Study the drawing (mm; zero at the part's minimum x, y, z) and answer. Round coordinates to 2 decimals unless told otherwise and drop trailing zeros. Write each loop counter-clockwise with the first axis right and the second up, starting at its lowest first coordinate (ties: lowest second). Pieces come first, ordered by that corner, then holes. Notation, with made-up numbers: (58.25, 75) -> (73.25, 75) arc R5 ccw to (73.25, 79) -> close; hole circle Ø4 at (63, 84.25). An arc over 180 degrees is marked (long way). Return JSON: item names as keys, results as strings.
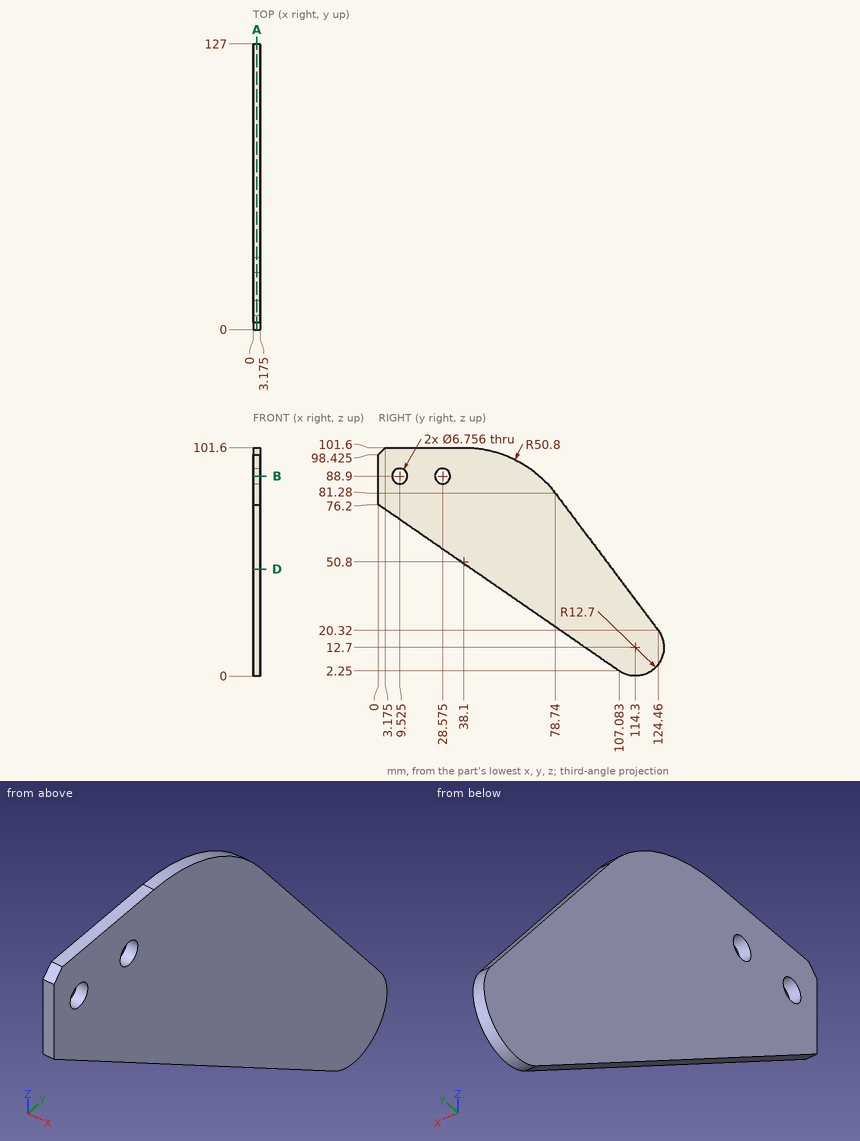
Item 1: Section A-A (x = 1.7) is taken. State how many separate pieces and enclosed holes the cut face has, then the cut area to 3 significant figures.
Worked answers:
{"separate pieces": "1", "enclosed holes": "2", "area": "5,800 mm2"}
Item 2: Straight lines are drawn through the part: L1, parallel to Y at x = 2.1, z = 88.9 (1 decimal); L2, parallel to Y at x = 2.5, z = 88.5; L3, parallel to Z at x = 1.6, y = 9 (1 decimal). For each, find the intervals that lie inside material, in ascending order. Write a range as [from, to].
Worked answers:
{"L1": "y = [0, 6.1], [12.9, 25.2], [32, 71.7]", "L2": "y = [0, 6.17], [12.88, 25.22], [31.93, 72.15]", "L3": "z = [70, 85.6], [92.2, 101.6]"}
Item 3: Section B-B (z = 88.9) is taken. Give the vertices of the cut face in (x, y) (1 decimal), then the cut area to 3 significant figures.
Worked answers:
{"outline": "(0, 0) -> (3.2, 0) -> (3.2, 6.1) -> (0, 6.1) -> close; (0, 12.9) -> (3.2, 12.9) -> (3.2, 25.2) -> (0, 25.2) -> close; (0, 32) -> (3.2, 32) -> (3.2, 71.7) -> (0, 71.7) -> close", "area": "185 mm2"}
Item 4: Flat-ended cylindrical pins translate along their axes: pin 1 (9 mm diameter, centred on y = 9.525, z = 88.9, fed in from -X); pin 2 (1 mm diameter, centred on x = 2.5, y = 44, fed in from -Z); pin 3 (1 mm diameter, centred on x = 0.5, y = 70.5, fed in from -Z). Find the tip coordinate at first contact, or state that the pin passes through.
Worked answers:
{"pin 1": "stops at x = 0", "pin 2": "stops at z = 45.47", "pin 3": "stops at z = 27.17"}
Item 5: Section D-D (z = 47.5) is taken. Give the vertices of the cut face in (x, y) (1 decimal).
Worked answers:
{"outline": "(0, 41.6) -> (3.2, 41.6) -> (3.2, 104.1) -> (0, 104.1) -> close"}
